Geometry: final body of the model. Coordinates: model frame, mm. A direction names the side the tool comes from. Round coordinates to 2 decimals unless told otherwise and drop trailing zeros. Loops run counter-clockwise (first coordinate to the right, second up) from the corner with the lowest first, then second, coordinate; pieces in that order, holes last. Notation, with made-up numbers: M 13.5,59 L 40.5,59 A24 ccw 40.5,86 Z; hole C 87.25,49 d7. An arc over 180 degrees is marked long. Write each question's results on one line, items separated by ' | '.
```python
from build123d import *

# Parameters (mm, degrees)
F1_DEPTH = 2
F2_W     = 46
F2_H     = 49
F3_DEPTH = 22
F4_W     = 42
F4_H     = 45
F5_DEPTH = 20
F6_R     = 4
F7_R     = 2
F8_R     = 2
F9_R     = 4


with BuildPart() as f1:
    # F0 (on Top) → F1 (new body)
    with BuildSketch(Plane.XY):
        with BuildLine():
            Line((7, 10), (-7, 10))
            ThreePointArc((-7, 10), (-9.1213203436, 9.1213203436), (-10, 7))
            Line((-10, 7), (-10, -7))
            ThreePointArc((-10, -7), (-9.1213203436, -9.1213203436), (-7, -10))
            Line((-7, -10), (7, -10))
            ThreePointArc((7, -10), (9.1213203436, -9.1213203436), (10, -7))
            Line((10, -7), (10, 7))
            ThreePointArc((10, 7), (9.1213203436, 9.1213203436), (7, 10))
        make_face()
    extrude(amount=F1_DEPTH)

    # F2 (on face) → F3 (join)
    with BuildSketch(Plane.XY.offset(2)):
        Rectangle(F2_W, F2_H)
        with BuildLine():
            Line((-7, 10), (7, 10))
            ThreePointArc((7, 10), (9.1213203436, 9.1213203436), (10, 7))
            Line((10, 7), (10, -7))
            ThreePointArc((10, -7), (9.1213203436, -9.1213203436), (7, -10))
            Line((7, -10), (-7, -10))
            ThreePointArc((-7, -10), (-9.1213203436, -9.1213203436), (-10, -7))
            Line((-10, -7), (-10, 7))
            ThreePointArc((-10, 7), (-9.1213203436, 9.1213203436), (-7, 10))
        make_face(mode=Mode.SUBTRACT)
        with BuildLine():
            ThreePointArc((10, 7), (9.1213203436, 9.1213203436), (7, 10))
            Line((7, 10), (-7, 10))
            ThreePointArc((-7, 10), (-9.1213203436, 9.1213203436), (-10, 7))
            Line((-10, 7), (-10, -7))
            ThreePointArc((-10, -7), (-9.1213203436, -9.1213203436), (-7, -10))
            Line((-7, -10), (7, -10))
            ThreePointArc((7, -10), (9.1213203436, -9.1213203436), (10, -7))
            Line((10, -7), (10, 7))
        make_face()
    extrude(amount=F3_DEPTH)

    # F4 (on face) → F5 (cut)
    with BuildSketch(Plane.XY.offset(24)):
        Rectangle(F4_W, F4_H)
    extrude(amount=-F5_DEPTH, mode=Mode.SUBTRACT)

    # F6
    f6_edges = [f1.edges().sort_by_distance(p)[0] for p in [
        (-23, 24.5, 13),
        (23, 24.5, 13),
        (23, -24.5, 13),
        (-23, -24.5, 13),
    ]]
    fillet(f6_edges, radius=F6_R)

    # F7
    f7_edges = [f1.edges().sort_by_distance(p)[0] for p in [
        (21, 22.5, 14),
        (21, -22.5, 14),
        (-21, -22.5, 14),
        (-21, 22.5, 14),
    ]]
    fillet(f7_edges, radius=F7_R)

    # F8
    f8_edges = [f1.edges().sort_by_distance(p)[0] for p in [
        (0, 22.5, 4),
        (20.414214, 21.914214, 4),
        (-20.414214, 21.914214, 4),
        (21, 0, 4),
        (-21, 0, 4),
        (20.414214, -21.914214, 4),
        (-20.414214, -21.914214, 4),
        (0, -22.5, 4),
    ]]
    fillet(f8_edges, radius=F8_R)

    # F9
    f9_edges = [f1.edges().sort_by_distance(p)[0] for p in [
        (0, 24.5, 2),
        (-21.828427, 23.328427, 2),
        (-23, 0, 2),
        (-21.828427, -23.328427, 2),
        (0, -24.5, 2),
        (21.828427, -23.328427, 2),
        (23, 0, 2),
        (21.828427, 23.328427, 2),
    ]]
    fillet(f9_edges, radius=F9_R)


solid = f1.part
```
1. Section D-D (z = 3.25). Output: boundary loops of the cut face in (x, y), then the cut area to 3 significant figures.
Answer key:
outline: M -21.9,-20.5 A2.9 ccw -19,-23.4 L 19,-23.4 A2.9 ccw 21.9,-20.5 L 21.9,20.5 A2.9 ccw 19,23.4 L -19,23.4 A2.9 ccw -21.9,20.5 Z | area: 2,040 mm²
2. Ray query, probe 1 along Y at (x, z) = (-16, 11); probe 2 along X at (y, z) = (7.5, 12.5); probe 3 along Z at (x, y) = (16, -3.5). Return the intervals inside material, ascending.
Answer key:
probe 1: y = -24.5 to -22.5, 22.5 to 24.5 | probe 2: x = -23 to -21, 21 to 23 | probe 3: z = 2 to 4
3. Draft query along Y for faces 1 (the face through (20.43, -0.29, 4.6)), 2 (the face through (21.797, -23.359, 15.126)), 3 (the face through (-10, 0, 1)). Return one class per face: pulls with the +Y half, pulls with the -Y half, needs draft (parallel to the pull), parting line crosses it, or undercut.
Answer key:
face 1: undercut | face 2: pulls with the -Y half | face 3: needs draft
4. Section C-C (x = 11.5). Output: boundary loops of the cut face in (y, z), then the cut area to 3 significant figures.
Answer key:
outline: M -24.5,6 A4 ccw -20.5,2 L 20.5,2 A4 ccw 24.5,6 L 24.5,24 L 22.5,24 L 22.5,6 A2 cw 20.5,4 L -20.5,4 A2 cw -22.5,6 L -22.5,24 L -24.5,24 Z | area: 173 mm²
5. Section A-A (z = 13). Output: boundary loops of the cut face in (x, y).
Answer key:
outline: M -23,-20.5 A4 ccw -19,-24.5 L 19,-24.5 A4 ccw 23,-20.5 L 23,20.5 A4 ccw 19,24.5 L -19,24.5 A4 ccw -23,20.5 Z; hole M -21,-20.5 A2 ccw -19,-22.5 L 19,-22.5 A2 ccw 21,-20.5 L 21,20.5 A2 ccw 19,22.5 L -19,22.5 A2 ccw -21,20.5 Z
6. Pin query (flat end, axial travel): P1, Ø12, axis at x = -7.5, y = -14.5, coming from the -Z side; P2, Ø1.6, axis at x = 1.5, z = 1, coming from the +Y side; P3, Ø1.6, axis at y = -3.5, z = 1, coming from the -X side; P4, Ø1.6, axis at y = -1, z = 1, coming from the +X side. Return the tip coordinate at first contact, or that it passes through.
Answer key:
P1: stops at z = 0 | P2: stops at y = 10 | P3: stops at x = -10 | P4: stops at x = 10
7. Section B-B (y = -15.5). Output: boundary loops of the cut face in (x, z).
Answer key:
outline: M -23,6 A4 ccw -19,2 L 19,2 A4 ccw 23,6 L 23,24 L 21,24 L 21,6 A2 cw 19,4 L -19,4 A2 cw -21,6 L -21,24 L -23,24 Z
8. Access query for faces 4 (the face through (9.14, 9.1, 0.99)), 5 (the face through (-20.4, 21.93, 14.87)), 6 (the face through (0, -10, 1)). Directions: +Z, -Z, +X, -X, +Y, -Y. A direction counts if a zero-diameter tool reaches every point of the face in a straight line with its end or side. Return the directions, or none.
Answer key:
face 4: -Z, +X, +Y | face 5: +Z | face 6: -Z, +X, -X, -Y
